```python
from build123d import *

# Parameters (mm, degrees)
SKETCH_1_W      = 100
SKETCH_1_H      = 30
EXTRUDE_3_DEPTH = 25


with BuildPart() as part:
    # 草图1 → 凸台-拉伸3 (new body)
    with BuildSketch(Plane(origin=(0, 0, 0), x_dir=(1, 0, 0), z_dir=(0, 1, 0))):
        Rectangle(SKETCH_1_W, SKETCH_1_H)
        with BuildLine():
            ThreePointArc((39.834535229, 8.75370031), (43.612356016, 5.082059017), (45, 0))
            ThreePointArc((45, 0), (43.620805853, -5.067712151), (39.863658712, -8.737552514))
            ThreePointArc((39.863658712, -8.737552514), (34.79927033, -14.006397834), (29.887949458, -8.594587789))
            ThreePointArc((29.887949458, -8.594587789), (25, 0), (29.887949458, 8.594587789))
            ThreePointArc((29.887949458, 8.594587789), (34.773112936, 14.183369273), (39.834535229, 8.75370031))
        make_face(mode=Mode.SUBTRACT)
    extrude(amount=EXTRUDE_3_DEPTH)


solid = part.part
```
The listing builds one solid part. Answer for the finished solid, in the listing's coordinates (mm). Round coordinates to 2 decimals unless told otherwise and drop trailing zeros. Loops run counter-clockwise (first coordinate to the right, second up) from the corner with the lowest first, then second, coordinate; pieces in that order, holes last. Notation, with made-up numbers: (43.25, 73.5) -> (88.25, 73.5) arc R24 cw to (88.25, 100.5) -> close; hole circle Ø10 at (69, -38.5). An arc over 180 degrees is marked (long way). Use one line per item in the form item = value.
1. A flat-ended cylindrical pin translates along its axis: pin 1 Ø1.5 at (x, z) = (17, -11) entering from -Y. Find the tip coordinate at first contact, or state that the pin passes through.
Answer key:
pin_1 = 0
2. For a pull along Z with two mould halves and no side action, classify faces 1 (the flat face through (-1, 12, -15)), 2 (the flat face through (-50, 12, 0)), 3 (the flat face through (-1, 12, 15)), 4 (the cylindrical face through (25, 12, 0)) as released by +Z, released by -Z, zero draft, split by the parting line, or undercut.
Answer key:
face_1 = released by -Z
face_2 = zero draft
face_3 = released by +Z
face_4 = undercut
3. The part is cut by section B-B on z = -3.5. Determine the outline of the cut face in (x, y).
Answer key:
outline = (-50, 0) -> (25.63, 0) -> (25.63, 25) -> (-50, 25) -> close; (44.37, 0) -> (50, 0) -> (50, 25) -> (44.37, 25) -> close
4. The part is cut by section C-C on y = 1.75. Determine the outline of the cut face in (x, z).
Answer key:
outline = (-50, -15) -> (50, -15) -> (50, 15) -> (-50, 15) -> close; hole (29.89, -8.59) arc R5 ccw (long way) to (39.83, -8.75) arc R10 ccw to (39.86, 8.74) arc R5 ccw (long way) to (29.89, 8.59) arc R10 ccw to start
5. Find the intervals of material crossed by probe 1 along X at (y, z) = (3, -1.5); probe 2 along X at (y, z) = (23, 10.75); probe 3 along Z at (x, y) = (35.5, 10.25), in increasing order. Write a range as [from, to].
Answer key:
probe_1 = [-50, 25.11], [44.89, 50]
probe_2 = [-50, 30.18], [39.56, 50]
probe_3 = [-15, -14.14], [13.97, 15]
6. The part is cut by section A-A on x = 27. Determine the outline of the cut face in (y, z), and give its area (3 significant figures).
Answer key:
outline = (0, -15) -> (25, -15) -> (25, -6) -> (0, -6) -> close; (0, 6) -> (25, 6) -> (25, 15) -> (0, 15) -> close
area = 450 mm²
